```python
from build123d import *

# Parameters (mm, degrees)
F1_DEPTH = 3
F2_R     = 8
F2_R_2   = 1.1
F3_DEPTH = 25


with BuildPart() as f1:
    # F0 (on Front) → F1 (new body)
    with BuildSketch(Plane.XZ):
        with BuildLine():
            ThreePointArc((0, 5), (1.464466, 1.464466), (5, 0))
            Line((5, 0), (230.7, 0))
            ThreePointArc((230.7, 0), (234.235534, 1.464466), (235.7, 5))
            Line((235.7, 5), (235.7, 50.3))
            ThreePointArc((235.7, 50.3), (234.235534, 53.835534), (230.7, 55.3))
            Line((230.7, 55.3), (5, 55.3))
            ThreePointArc((5, 55.3), (1.464466, 53.835534), (0, 50.3))
            Line((0, 50.3), (0, 5))
        make_face()
    extrude(amount=F1_DEPTH)

    # F2 (on face) → F3 (cut)
    with BuildSketch(Plane.XZ.offset(3)):
        with Locations((13.5, 15)):
            Circle(F2_R)
        with Locations((13.5, 40)):
            Circle(F2_R)
        with Locations((32.5, 15)):
            Circle(F2_R)
        with Locations((32.5, 40)):
            Circle(F2_R)
        with Locations((51.5, 15)):
            Circle(F2_R)
        with Locations((51.5, 40)):
            Circle(F2_R)
        with Locations((70.5, 15)):
            Circle(F2_R)
        with Locations((70.5, 40)):
            Circle(F2_R)
        with Locations((89.5, 15)):
            Circle(F2_R)
        with Locations((89.5, 40)):
            Circle(F2_R)
        with Locations((108.5, 15)):
            Circle(F2_R)
        with Locations((108.5, 40)):
            Circle(F2_R)
        with Locations((127.5, 15)):
            Circle(F2_R)
        with Locations((127.5, 40)):
            Circle(F2_R)
        with Locations((146.5, 15)):
            Circle(F2_R)
        with Locations((146.5, 40)):
            Circle(F2_R)
        with Locations((165.5, 15)):
            Circle(F2_R)
        with Locations((165.5, 40)):
            Circle(F2_R)
        with Locations((184.5, 15)):
            Circle(F2_R)
        with Locations((184.5, 40)):
            Circle(F2_R)
        with Locations((203.5, 15)):
            Circle(F2_R)
        with Locations((203.5, 40)):
            Circle(F2_R)
        with Locations((222.5, 15)):
            Circle(F2_R)
        with Locations((222.5, 40)):
            Circle(F2_R)
        with Locations((7, 27.65)):
            Circle(F2_R_2)
        with Locations((228.7, 27.65)):
            Circle(F2_R_2)
    extrude(amount=-F3_DEPTH, mode=Mode.SUBTRACT)


solid = f1.part
```
Part model, mm, in its own coordinate system. Give positions to 0.01 mm unless a question says otherwise; leave off trailing zeros. Loops run counter-clockwise (first coordinate to the right, second up) from the corner with the lowest first, then second, coordinate; pieces in that order, holes last. Notation, with made-up numbers: M 43,16.25 L 81,16.25 A19 cw 81,33.25 Z; hole C 61.25,39.5 d1. An arc over 180 degrees is marked long. Return JSON: item names as keys, results as strings.
1) Drill centre lines: line 1 (Z direction, x = 165.5, y = -0.7); line 2 (Z direction, x = 197.5, y = -1.2); line 3 (Z direction, x = 7, y = -1.95). Where is each one in solid material? Low to high.
Calculated:
{"line 1": "z = 0 to 7, 23 to 32, 48 to 55.3", "line 2": "z = 0 to 9.71, 20.29 to 34.71, 45.29 to 55.3", "line 3": "z = 0 to 10.34, 19.66 to 26.55, 28.75 to 35.34, 44.66 to 55.3"}
2) Saw through at D-D, the plane x = 152.5. List the corners of the cut face in (y, z).
Calculated:
{"outline": "M -3,0 L 0,0 L 0,9.71 L -3,9.71 Z; M -3,20.29 L 0,20.29 L 0,34.71 L -3,34.71 Z; M -3,45.29 L 0,45.29 L 0,55.3 L -3,55.3 Z"}
3) Saw through at A-A, the plane y = -0.55. Count the separate pieces of the cut face and the enclosed holes in it, then the cut area to 3 significant figures.
Calculated:
{"separate pieces": "1", "enclosed holes": "26", "area": "8,180 mm2"}
4) Flat gauge pins, fed straight in: pin 1 Ø14.5 at (x, z) = (108.5, 40) entering from +Y; pin 2 Ø3 at (x, z) = (88.5, 33) entering from +Y. Where does each tip first touch, or does it go through?
Calculated:
{"pin 1": "passes through", "pin 2": "stops at y = 0"}
5) Saw through at B-B, the plane x = 32.5. List the corners of the cut face in (y, z).
Calculated:
{"outline": "M -3,0 L 0,0 L 0,7 L -3,7 Z; M -3,23 L 0,23 L 0,32 L -3,32 Z; M -3,48 L 0,48 L 0,55.3 L -3,55.3 Z"}
6) Pull direction Z, two halves, no side cores. Call faces 1 (the face through (234.2, -1.48, 1.43)), 2 (the face through (116, -3, 28)), 3 (the face through (216.6, -1.5, 45.4)), 4 (the face through (64.6, -1.5, 45.4)): released by +Z, released by -Z, zero draft, split by the parting line, or undercut.
Calculated:
{"face 1": "released by -Z", "face 2": "zero draft", "face 3": "undercut", "face 4": "undercut"}
